Model file for the job. Use its own axes, mm. A direction names the side the tool comes from. Give positions to 0.01 mm unless a question says otherwise; leave off trailing zeros. Write each loop counter-clockwise with the first axis right and the second up, starting at its lowest first coordinate (ties: lowest second). Pieces come first, ordered by that corner, then holes.
```python
from build123d import *

# Parameters (mm, degrees)
SKETCH1_R           = 63.5
BOSS_EXTRUDE1_DEPTH = 76.2
SKETCH2_R           = 57.15
CUT_EXTRUDE1_DEPTH  = 73.025
SKETCH3_R           = 60.325
CUT_EXTRUDE2_DEPTH  = 25.4


with BuildPart() as part:
    # Sketch1 → Boss-Extrude1 (new body)
    with BuildSketch(Plane(origin=(0, 0, 0), x_dir=(1, 0, 0), z_dir=(0, 1, 0))):
        with Locations(Location((0, 0, 0), (0, 0, 90))):
            Circle(SKETCH1_R)
    extrude(amount=BOSS_EXTRUDE1_DEPTH)

    # Sketch2 → Cut-Extrude1 (cut)
    with BuildSketch(Plane(origin=(0, 76.2, 0), x_dir=(1, 0, 0), z_dir=(0, 1, 0))):
        with Locations(Location((0, 0, 0), (0, 0, 270))):
            Circle(SKETCH2_R)
    extrude(amount=-CUT_EXTRUDE1_DEPTH, mode=Mode.SUBTRACT)

    # Sketch3 → Cut-Extrude2 (cut)
    with BuildSketch(Plane(origin=(0, 76.2, 0), x_dir=(1, 0, 0), z_dir=(0, 1, 0))):
        with Locations(Location((0, 0, 0), (0, 0, 270))):
            Circle(SKETCH3_R)
    extrude(amount=-CUT_EXTRUDE2_DEPTH, mode=Mode.SUBTRACT)


solid = part.part
```
1. Pull direction Z, two halves, no side cores. Call faces 3 (the flat face through (23, 76.2, -56)), 4 (the cylindrical face through (61.99, 37.57, 13.77)), 5 (the cylindrical face through (2.513, 27.321, -57.095)): +Z half, -Z half, draft (parallel to the pull), parting line (faces both ways), or undercut.
Calculated:
face 3: draft
face 4: parting line
face 5: undercut
2. Slice it at A-A, the plane x = 0. Write the cut outline in (y, z) (3 decimals).
Calculated:
outline: (0, -63.5) - (76.2, -63.5) - (76.2, -60.325) - (50.8, -60.325) - (50.8, -57.15) - (3.175, -57.15) - (3.175, 57.15) - (50.8, 57.15) - (50.8, 60.325) - (76.2, 60.325) - (76.2, 63.5) - (0, 63.5) - close
3. Slice it at B-B, the plane y = 6.5. Write the cut outline in (x, z).
Calculated:
outline: circle Ø127 at (0, 0); hole circle Ø114.3 at (0, 0)
4. Slice it at C-C, the plane z = 0. Write the cut outline in (x, y) (3 decimals), and give its area (3 significant figures).
Calculated:
outline: (-63.5, 0) - (63.5, 0) - (63.5, 76.2) - (60.325, 76.2) - (60.325, 50.8) - (57.15, 50.8) - (57.15, 3.175) - (-57.15, 3.175) - (-57.15, 50.8) - (-60.325, 50.8) - (-60.325, 76.2) - (-63.5, 76.2) - close
area: 1,170 mm2
5. Which spindle directions (+Z, -Z, +X, -X, +Y, -Y) get a long thin tool onto all of the face, cutting with end or side? Do faces 1 (the cylindrical face through (2.652, 63.678, -60.267)), 2 (the flat face through (-1, 0, 1)). Say none if no direction does.
Calculated:
face 1: +Y
face 2: +Z, -Z, +X, -X, -Y
6. Pin check, flat tips, straight feed: P1, Ø1.5, axis at y = 61.5, z = -12, coming from the -X side; P2, Ø2, axis at x = 45, z = 5, coming from the +Y side (3 decimals); P3, Ø2, axis at x = 50.5, y = 44.5, coming from the +Z side. Stop position of each tip, or through.
Calculated:
P1: stops at x = -62.5
P2: stops at y = 3.175
P3: stops at z = 39.77
7. Probe probe 1 along X at (y, z) = (67.25, 0) (3 decimals); probe 2 along X at (y, z) = (21, 0); probe 3 along Y at (x, z) = (-38.5, -16.5) (3 decimals). List the from-to ranges inside material, lowest first.
Calculated:
probe 1: x = -63.5 to -60.325, 60.325 to 63.5
probe 2: x = -63.5 to -57.15, 57.15 to 63.5
probe 3: y = 0 to 3.175
